CAD build for the part. Positions are in the model's coordinates, mm. A direction names the side the tool comes from. Coordinates: 2 decimals unless noted, no trailing zeros. Write each loop counter-clockwise with the first axis right and the second up, starting at its lowest first coordinate (ties: lowest second). Pieces come first, ordered by that corner, then holes. Notation, with made-up numbers: (-14, 46) -> (34, 46) arc R20 ccw to (34, 73) -> close; hole circle Ø11 at (82, -20). An arc over 180 degrees is marked (long way). Answer as CSV lines item,"result".
```python
from build123d import *

# Parameters (mm, degrees)
F1_DEPTH = 96
F2_T     = -0.4
F3_W     = 25
F3_H     = 0.4
F4_DEPTH = 0.4
F6_DEPTH = 0.4
F5_W     = 6
F5_H     = 1
F7_DEPTH = 47


with BuildPart() as f1:
    # F0 (on Right) → F1 (new body)
    with BuildSketch(Plane.YZ):
        Polygon((0, 30), (0, 0), (47, 0), (47, 30), (0.4, 30), (0.4, 86), (0, 86), align=None)
    extrude(amount=-F1_DEPTH)

    # F2
    f2_openings = [f1.faces().sort_by_distance(p)[0] for p in [
        (-48, 23.5, 0),
    ]]
    offset(amount=F2_T, openings=f2_openings, kind=Kind.INTERSECTION)

    # F3 (on face) → F4 (cut, through all)
    with BuildSketch(Plane.XY.offset(30)):
        with BuildLine():
            ThreePointArc((-75.6825014059, 14.3409090909), (-68.5, 9), (-61.3174985941, 14.3409090909))
            ThreePointArc((-61.3174985941, 14.3409090909), (-58, 22), (-61.3174985941, 29.6590909091))
            ThreePointArc((-61.3174985941, 29.6590909091), (-68.5, 35), (-75.6825014059, 29.6590909091))
            ThreePointArc((-75.6825014059, 29.6590909091), (-79, 22), (-75.6825014059, 14.3409090909))
        make_face()
        with Locations((-68.5, 6.2)):
            Rectangle(F3_W, F3_H)
        Polygon((-51.2081224133, 38.2756121002), (-51, 38.6172040513), (-57.4902470714, 42.5715299044), (-56.1374513849, 44.7918775867), (-56.479043336, 45), (-58.0399614359, 42.4380603665), align=None)
        with BuildLine():
            ThreePointArc((-14.3174985941, 14.3409090909), (-11, 22), (-14.3174985941, 29.6590909091))
            ThreePointArc((-14.3174985941, 29.6590909091), (-21.5, 35), (-28.6825014059, 29.6590909091))
            ThreePointArc((-28.6825014059, 29.6590909091), (-32, 22), (-28.6825014059, 14.3409090909))
            ThreePointArc((-28.6825014059, 14.3409090909), (-21.5, 9), (-14.3174985941, 14.3409090909))
        make_face()
        with Locations((-21.5, 6.2)):
            Rectangle(F3_W, F3_H)
        Polygon((-11.0399614359, 42.4380603665), (-4.2081224133, 38.2756121002), (-4, 38.6172040513), (-10.4902470714, 42.5715299044), (-9.1374513849, 44.7918775867), (-9.479043336, 45), align=None)
    extrude(amount=-F4_DEPTH, mode=Mode.SUBTRACT)

    # F5 (on face) → F6 (cut, through all)
    with BuildSketch(Plane(origin=(0, 47, 0), x_dir=(-1, 0, 0), z_dir=(0, 1, 0))):
        with BuildLine():
            Line((17, 9), (26, 9))
            ThreePointArc((26, 9), (34, 17), (26, 25))
            Line((26, 25), (17, 25))
            ThreePointArc((17, 25), (9, 17), (17, 9))
        make_face()
        with BuildLine():
            Line((64, 9), (73, 9))
            ThreePointArc((73, 9), (81, 17), (73, 25))
            Line((73, 25), (64, 25))
            ThreePointArc((64, 25), (56, 17), (64, 9))
        make_face()
    extrude(amount=-F6_DEPTH, mode=Mode.SUBTRACT)

    # F5 (on face) → F7 (cut, through all)
    with BuildSketch(Plane(origin=(0, 47, 0), x_dir=(-1, 0, 0), z_dir=(0, 1, 0))):
        with Locations((21.5, 30.5)):
            Rectangle(F5_W, F5_H)
        with Locations((68.5, 30.5)):
            Rectangle(F5_W, F5_H)
    extrude(amount=-F7_DEPTH, mode=Mode.SUBTRACT)


solid = f1.part
```
Item 1: Saw through at D-D on x = -15.5. Give the cut face in (y, z), and give its area (3 significant figures).
Answer below:
outline,"(0, 0) -> (0.4, 0) -> (0.4, 29.6) -> (6, 29.6) -> (6, 30) -> (0.4, 30) -> (0.4, 86) -> (0, 86) -> close; (6.4, 29.6) -> (12, 29.6) -> (12, 30) -> (6.4, 30) -> close; (32, 29.6) -> (46.6, 29.6) -> (46.6, 24.86) -> (47, 24.86) -> (47, 30) -> (32, 30) -> close; (46.6, 0) -> (47, 0) -> (47, 9.14) -> (46.6, 9.14) -> close"
area,"50.4 mm2"
Item 2: Saw through at C-C on x = -68.5. Give the cut face in (y, z), and give its area (3 significant figures).
Answer below:
outline,"(0, 0) -> (0.4, 0) -> (0.4, 29.6) -> (6, 29.6) -> (6, 30) -> (0, 30) -> close; (0, 31) -> (0.4, 31) -> (0.4, 86) -> (0, 86) -> close; (6.4, 29.6) -> (9, 29.6) -> (9, 30) -> (6.4, 30) -> close; (35, 29.6) -> (46.6, 29.6) -> (46.6, 25) -> (47, 25) -> (47, 30) -> (35, 30) -> close; (46.6, 0) -> (47, 0) -> (47, 9) -> (46.6, 9) -> close"
area,"47.5 mm2"
Item 3: Saw through at B-B on z = 17. Give the cut face in (x, y).
Answer below:
outline,"(-96, 0) -> (0, 0) -> (0, 47) -> (-9, 47) -> (-9, 46.6) -> (-0.4, 46.6) -> (-0.4, 0.4) -> (-95.6, 0.4) -> (-95.6, 46.6) -> (-81, 46.6) -> (-81, 47) -> (-96, 47) -> close; (-56, 46.6) -> (-34, 46.6) -> (-34, 47) -> (-56, 47) -> close"
Item 4: Saw through at A-A on y = 10.5. Give the cut face in (x, z).
Answer below:
outline,"(-96, 0) -> (-95.6, 0) -> (-95.6, 29.6) -> (-73, 29.6) -> (-73, 30) -> (-96, 30) -> close; (-64, 29.6) -> (-26, 29.6) -> (-26, 30) -> (-64, 30) -> close; (-17, 29.6) -> (-0.4, 29.6) -> (-0.4, 0) -> (0, 0) -> (0, 30) -> (-17, 30) -> close"
Item 5: Wall check: line 1 (X direction, y = 5, z = 13.5); line 2 (Y direction, x = -6, z = 57.5); line 3 (Y direction, x = -28.5, z = 27.5). Give the ranges that are in metal, low to high. Write a range as from..to.
Answer below:
line 1,"x = -96..-95.6, -0.4..0"
line 2,"y = 0..0.4"
line 3,"y = 0..0.4, 46.6..47"
Item 6: 3-axis set-ups, long thin cutter, end or side, ignore diameter. For faces 4 (the flat face through (-54.672, 40.386, 29.803)), 5 (the cylindrical face through (-80.998, 46.803, 16.824)), 6 (the flat face through (-0.4, 23, 15)): which of +Z, -Z, +X, -X, +Y, -Y reach the whole face in a straight line?
Answer below:
face 4,"+Z, -Z"
face 5,"+Y"
face 6,"-Z"
Item 7: Flat gauge pins, fed straight in: pin 1 (2 mm diameter, centred on x = -40.5, z = 40.5, fed in from +Y); pin 2 (10 mm diameter, centred on x = -78, y = 11, fed in from +Z); pin 3 (1 mm diameter, centred on x = -35, y = 16, fed in from -Z). Where does each tip first touch, or does it go through?
Answer below:
pin 1,"stops at y = 0.4"
pin 2,"stops at z = 30"
pin 3,"stops at z = 29.6"
Item 8: Two-plate mould, pull along Y, no slides. Class faces 1 (the flat face through (-47, 47, 15)), 2 (the flat face through (-47, 24, 30)), 3 (the flat face through (-54.2, 40.567, 29.803)): pulls with the +Y half, pulls with the -Y half, needs draft (parallel to the pull), parting line crosses it, or undercut.
Answer below:
face 1,"pulls with the +Y half"
face 2,"needs draft"
face 3,"undercut"
